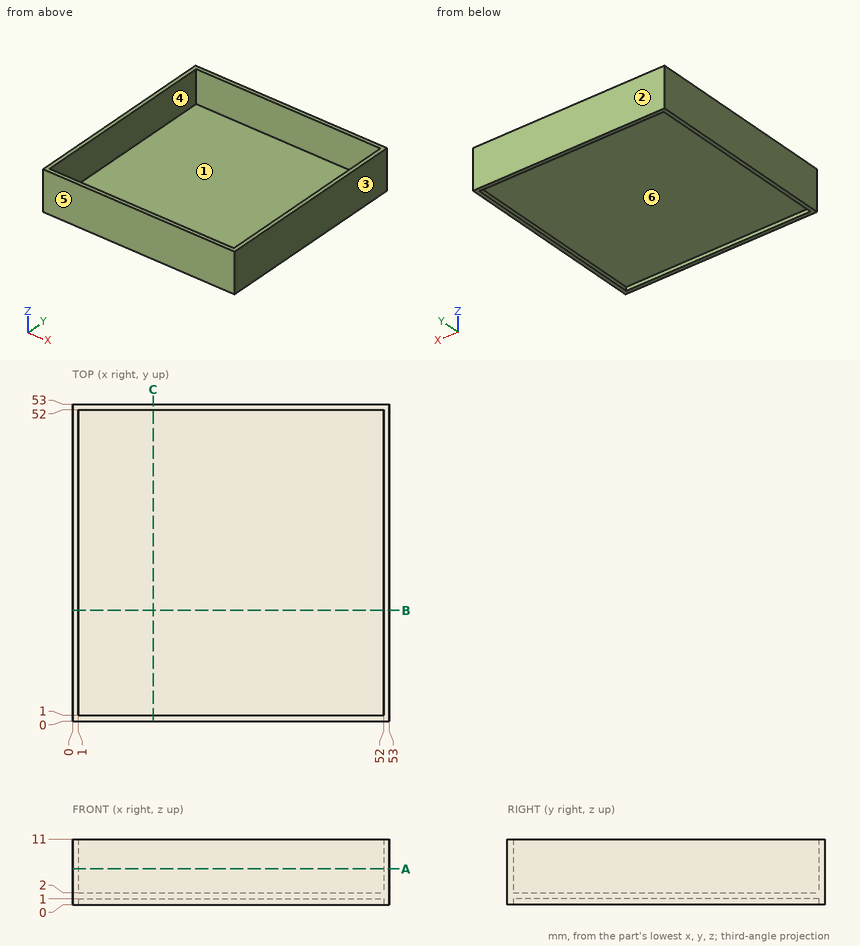
Design review of the part shown in the three views and the two pictorial views. Dimensions are in mm from the part's minimum x, y and z. A direction names the side the tool comes from. Round coordinates to 2 decimals unless told otherwise and drop trailing zeros. Order: outer loops, then holes, each group sorted by start corner. A loop starts at its lowest first (then second) coordinate and runs counter-clockwise, first axis right, second up. Notation, with made-up numbers: (-1.5, -2.75) - (15.5, -2.75) arc R15 ccw to (15.5, 6.25) - close; hole circle Ø5 at (-35.75, 72). An arc over 180 degrees is marked (long way). Answer in a Markdown table with one row per item.
(1) Machinability: for the marked faces 4, 5 and 6, which of the approach directions +Z, -Z, +X, -X, +Y, -Y give a long, thin tool a straight path to every point of the face, cutting with its end or side? Answer none if there is none.
Result set:
| item | result |
|---|---|
| face 4 | +Z |
| face 5 | +Z, -Z, +X, -X, -Y |
| face 6 | -Z |
(2) Mouldability with a two-part tool opening along X and no side actions: class the marked faces 1, 2 and 3 as released by +X, released by -X, zero draft, split by the parting line, or undercut.
Result set:
| item | result |
|---|---|
| face 1 | undercut |
| face 2 | zero draft |
| face 3 | released by +X |
(3) Take a section at A-A on z = 6. Write out the cut boundary in (x, y), plus the area to 3 significant figures.
Result set:
| item | result |
|---|---|
| outline | (0, 0) - (53, 0) - (53, 53) - (0, 53) - close; hole (1, 1) - (52, 1) - (52, 52) - (1, 52) - close |
| area | 208 mm2 |
(4) Take a section at B-B on y = 18.5. Write out the cut boundary in (x, z).
Result set:
| item | result |
|---|---|
| outline | (0, 0) - (1, 0) - (1, 1) - (52, 1) - (52, 0) - (53, 0) - (53, 11) - (52, 11) - (52, 2) - (1, 2) - (1, 11) - (0, 11) - close |
(5) Clearance check with a flat-ended pin moving along its axis: P1, Ø15.5, axis at x = 24.5, y = 35, coming from the +Z side. State where the tip first meets the part, or that it passes through.
Result set:
| item | result |
|---|---|
| P1 | stops at z = 2 |
(6) For line 1 (Y direction, x = 16, z = 3.5); line 2 (Z direction, x = 38, y = 39.5), list the stretches that pass through material, from the lowest coordinate up. Write a range as from..to.
Result set:
| item | result |
|---|---|
| line 1 | y = 0..1, 52..53 |
| line 2 | z = 1..2 |
